Check sheet for the modelled part. Datum: model origin and axes. Units: mm. Face numbers are marked on the shaded views. Round coordinates to 2 decimals unless told otherwise and drop trailing zeros. Order: outer loops, then holes, each group sorted by start corner. A loop starts at its lowest first (then second) coordinate and runs counter-clockwise, first axis right, second up.
```python
from build123d import *

# Parameters (mm, degrees)
BOSS_EXTRUDE1_DEPTH = 67
SKETCH2_R           = 20
CUT_EXTRUDE1_DEPTH  = 1.5
BOSS_EXTRUDE3_DEPTH = 1.5
SKETCH8_R           = 3.15
CUT_EXTRUDE2_DEPTH  = 12.5


with BuildPart() as part:
    # Sketch1 → Boss-Extrude1 (new body)
    with BuildSketch(Plane(origin=(0, 0, 0), x_dir=(0, 0, -1), z_dir=(1, 0, 0))):
        with BuildLine():
            Line((0, 70), (-50, 70))
            Line((-50, 70), (-50, 0))
            Line((-50, 0), (0, 0))
            Line((0, 0), (0, 17.5))
            Line((0, 17.5), (-6.545517328, 17.5))
            ThreePointArc((-6.545517328, 17.5), (-42, 27), (-6.545517328, 36.5))
            Line((-6.545517328, 36.5), (0, 36.5))
            Line((0, 36.5), (0, 54.2))
            Line((0, 54.2), (-29, 54.2))
            Line((-29, 54.2), (-29, 57.5))
            Line((-29, 57.5), (0, 57.5))
            Line((0, 57.5), (0, 70))
        make_face()
    extrude(amount=-BOSS_EXTRUDE1_DEPTH)

    # Sketch2 → Cut-Extrude1 (cut)
    with BuildSketch(Plane(origin=(-12.5, 0, 0), x_dir=(0, 0, -1), z_dir=(1, 0, 0))):
        with Locations((-23, 27)):
            Circle(SKETCH2_R)
    cut_extrude1 = extrude(amount=CUT_EXTRUDE1_DEPTH, mode=Mode.SUBTRACT)

    # Mirror1: Cut-Extrude1 across plane
    add(cut_extrude1.mirror(Plane(origin=(-33.5, 0, 0), x_dir=(0, 0, 1), z_dir=(1, 0, 0))), mode=Mode.SUBTRACT)

    # Sketch7 → Boss-Extrude3 (add)
    with BuildSketch(Plane.XY.offset(50)):
        Polygon((-60.553250223, 0), (-6.967587392, 0), (-33.650176709, 28.153479174), align=None)
        Polygon((0, 6.603562983), (0, 63.367654561), (-27.0098942, 35.102389871), align=None)
        Polygon((-67, 63.341726624), (-67, 7.149153864), (-40.262049953, 35.129834934), align=None)
        Polygon((-6.940604727, 70), (-60.084264634, 70), (-33.621767444, 42.078745631), align=None)
    extrude(amount=BOSS_EXTRUDE3_DEPTH)

    # Sketch8 → Cut-Extrude2 (cut)
    with BuildSketch(Plane(origin=(0, 70, 0), x_dir=(1, 0, 0), z_dir=(0, 1, 0))):
        with Locations((-33.5, -8.3)):
            Circle(SKETCH8_R)
    extrude(amount=-CUT_EXTRUDE2_DEPTH, mode=Mode.SUBTRACT)


solid = part.part
```
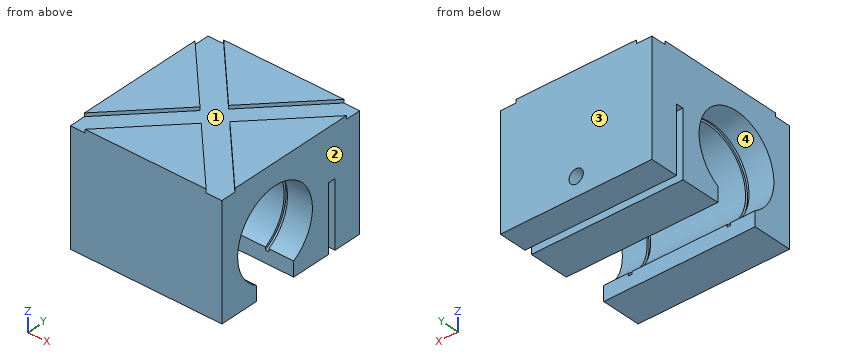
Item 1: Go/stop test with flat-tipped pins: P1, Ø1.6, axis at x = -17.5, y = 56.5, coming from the -Z side; P2, Ø5, axis at x = -51, y = 14, coming from the +Z side. Record where each tip stops, or that it passes through.
Answer:
P1: stops at z = 29
P2: stops at z = 50
Item 2: Sectioned sample at A-A (z = 23). Record the cut outline in (x, y).
Answer:
outline: (-67, 0) - (0, 0) - (0, 8) - (-11, 8) - (-11, 7) - (-12.5, 7) - (-12.5, 8) - (-54.5, 8) - (-54.5, 7) - (-56, 7) - (-56, 8) - (-67, 8) - close; (-67, 46) - (-56, 46) - (-56, 47) - (-54.5, 47) - (-54.5, 46) - (-12.5, 46) - (-12.5, 47) - (-11, 47) - (-11, 46) - (0, 46) - (0, 54.2) - (-67, 54.2) - close; (-67, 57.5) - (0, 57.5) - (0, 70) - (-67, 70) - close
Item 3: Sectioned sample at C-C (z = 39). Record the cut outline in (x, y), and give its area (3 significant figures).
Answer:
outline: (-67, 0) - (0, 0) - (0, 16.75) - (-11, 16.75) - (-11, 15) - (-12.5, 15) - (-12.5, 16.75) - (-54.5, 16.75) - (-54.5, 15) - (-56, 15) - (-56, 16.75) - (-67, 16.75) - close; (-67, 37.25) - (-56, 37.25) - (-56, 39) - (-54.5, 39) - (-54.5, 37.25) - (-12.5, 37.25) - (-12.5, 39) - (-11, 39) - (-11, 37.25) - (0, 37.25) - (0, 70) - (-67, 70) - close
area: 3,310 mm2
Item 4: Sectioned sample at B-B (z = 8.3). State how many separate pieces and enclosed holes the cut face has, and give its area (3 significant figures).
Answer:
separate pieces: 4
enclosed holes: 0
area: 2,770 mm2
Item 5: Release check for a two-part mould opening along Y. For the marked faces 1, 2, 3 and 4 record: released by +Y, released by -Y, zero draft, split by the parting line, or undercut.
Answer:
face 1: undercut
face 2: zero draft
face 3: released by +Y
face 4: undercut
Item 6: Sectioned sample at D-D (y = 27). Record the cut outline in (x, z).
Answer:
outline: (-67, 42) - (-56, 42) - (-56, 43) - (-54.5, 43) - (-54.5, 42) - (-12.5, 42) - (-12.5, 43) - (-11, 43) - (-11, 42) - (0, 42) - (0, 51.5) - (-19.33, 51.5) - (-19.33, 50) - (-32.56, 50) - (-32.56, 51.5) - (-34.75, 51.5) - (-34.75, 50) - (-48.03, 50) - (-48.03, 51.5) - (-67, 51.5) - close
Item 7: Scan lines: line 1 along Y through (x, z) = (-51.5, 23); line 2 along X through (y, z) = (64.5, 8.3); line 3 along Y through (x, z) = (-52, 12). Record each from-to range of solid material in increasing order.
Answer:
line 1: y = 0 to 8, 46 to 54.2, 57.5 to 70
line 2: x = -67 to -36.65, -30.35 to 0
line 3: y = 0 to 11.51, 42.49 to 54.2, 57.5 to 70
